```python
from build123d import *

# Parameters (mm, degrees)
SKETCH_1_W          = 260
SKETCH_1_H          = 300
EXTRUDE_1_DEPTH     = 10
SKETCH_2_W          = 220
SKETCH_2_H          = 260
CUT_EXTRUDE_1_DEPTH = 2
M3X0_51_D           = 2.5
M3X0_51_DEPTH       = 8.5
M3X0_51_TIP         = 0.751075774
SKETCH_9_W          = 260
SKETCH_9_H          = 300
SKETCH_9_W_2        = 240
SKETCH_9_H_2        = 280
CUT_EXTRUDE_3_DEPTH = 7
SKETCH_10_R         = 8
CUT_EXTRUDE_4_DEPTH = 11


with BuildPart() as part:
    # Эскиз1 → Бобышка-Вытянуть1 (new body)
    with BuildSketch(Plane(origin=(0, 0, 0), x_dir=(1, 0, 0), z_dir=(0, 1, 0))):
        Rectangle(SKETCH_1_W, SKETCH_1_H)
    extrude(amount=EXTRUDE_1_DEPTH)

    # Эскиз2 → Вырез-Вытянуть1 (cut)
    with BuildSketch(Plane.XZ):
        Rectangle(SKETCH_2_W, SKETCH_2_H)
    extrude(amount=-CUT_EXTRUDE_1_DEPTH, mode=Mode.SUBTRACT)

    # Отверстие обработанное метчиком M3x0.51
    with Locations(Plane(origin=(0, 0, 0), x_dir=(-1, 0, 0), z_dir=(0, -1, 0))):
        with Locations((-115, 135), (0, 135), (115, 135), (115, -135), (0, -135), (-115, -135), (115, 0), (-115, 0)):
            Hole(M3X0_51_D / 2, depth=M3X0_51_DEPTH)
            with Locations((0, 0, -(M3X0_51_DEPTH + M3X0_51_TIP / 2))):  # 118° drill point
                Cone(0, M3X0_51_D / 2, M3X0_51_TIP, mode=Mode.SUBTRACT)

    # Эскиз9 → Вырез-Вытянуть3 (cut)
    with BuildSketch(Plane.XZ):
        Rectangle(SKETCH_9_W, SKETCH_9_H)
        Rectangle(SKETCH_9_W_2, SKETCH_9_H_2, mode=Mode.SUBTRACT)
    extrude(amount=-CUT_EXTRUDE_3_DEPTH, mode=Mode.SUBTRACT)

    # Эскиз10 → Вырез-Вытянуть4 (cut, through all)
    with BuildSketch(Plane(origin=(0, 10, 0), x_dir=(1, 0, 0), z_dir=(0, 1, 0))):
        with Locations((74.221236429, -61.829520648)):
            Circle(SKETCH_10_R)
        with Locations((54.721236429, -61.829520648)):
            Circle(SKETCH_10_R)
        with Locations((35.221236429, -61.829520648)):
            Circle(SKETCH_10_R)
        with Locations((15.721236429, -61.829520648)):
            Circle(SKETCH_10_R)
        with Locations((-3.778763571, -61.829520648)):
            Circle(SKETCH_10_R)
        with Locations((-23.278763571, -61.829520648)):
            Circle(SKETCH_10_R)
        with Locations((-42.778763571, -61.829520648)):
            Circle(SKETCH_10_R)
        with Locations((-62.278763571, -61.829520648)):
            Circle(SKETCH_10_R)
        with Locations((27.756724611, -92.443317545)):
            Circle(SKETCH_10_R)
        with Locations((8.956724611, -92.443317545)):
            Circle(SKETCH_10_R)
        with Locations((-9.843275389, -92.443317545)):
            Circle(SKETCH_10_R)
        with Locations((-28.643275389, -92.443317545)):
            Circle(SKETCH_10_R)
        with Locations((40.197994593, -15.695954372)):
            Circle(SKETCH_10_R)
        with Locations((12.197994593, -15.695954372)):
            Circle(SKETCH_10_R)
        with Locations((-15.802005407, -15.695954372)):
            Circle(SKETCH_10_R)
        with Locations((-43.802005407, -15.695954372)):
            Circle(SKETCH_10_R)
        with Locations((64.84147229, 30.806375684)):
            Circle(SKETCH_10_R)
        with Locations((38.84147229, 30.806375684)):
            Circle(SKETCH_10_R)
        with Locations((12.84147229, 30.806375684)):
            Circle(SKETCH_10_R)
        with Locations((-13.15852771, 30.806375684)):
            Circle(SKETCH_10_R)
        with Locations((-39.15852771, 30.806375684)):
            Circle(SKETCH_10_R)
        with Locations((-65.15852771, 30.806375684)):
            Circle(SKETCH_10_R)
        with Locations((51.575799991, 106.283379385)):
            Circle(SKETCH_10_R)
        with Locations((25.075799991, 106.283379385)):
            Circle(SKETCH_10_R)
        with Locations((-1.424200009, 106.283379385)):
            Circle(SKETCH_10_R)
        with Locations((-27.924200009, 106.283379385)):
            Circle(SKETCH_10_R)
        with Locations((-0.103593652, 61.276056387)):
            Circle(SKETCH_10_R)
    extrude(amount=-CUT_EXTRUDE_4_DEPTH, mode=Mode.SUBTRACT)


solid = part.part
```
Can you work these out from the model? Positions are in its coordinate system, mm. A direction names the side the tool comes from. Round coordinates to 2 decimals unless told otherwise and drop trailing zeros. Loops run counter-clockwise (first coordinate to the right, second up) from the corner with the lowest first, then second, coordinate; pieces in that order, holes last. Notation, with made-up numbers: M 66.5,78.5 L 123.5,78.5 A12 cw 123.5,90.5 Z; hole C 61.25,14 d7. An arc over 180 degrees is marked long. Answer as a JSON object with one key per item and string values. Group by question number.
Q1. Imagine slicing it at C-C, the plane x = 94.5. Please give me the cut outline in (y, z).
Q2. Please list where these lines run through material, in increasing order: L1, parallel to Z at x = 115, y = 4.5; L2, parallel to X at y = 1, z = 80.5; L3, parallel to Z at x = -11, y = 2.75.
Q3. On a 3-axis mill with a long thin cutter (end or side, diameter ignored), from which of +Z, -Z, +X, -X, +Y, -Y can I reach the whole of each face in a straight line? I mean faces 4 (the flat face through (-2, 2, 2)), 5 (the cylindrical face through (49.842, 6.056, -98.474)). Say none if no direction works.
Q4. Will these pins go through, and if not, where does the flat tip stop? pin 1 (21 mm diameter, centred on x = 27.76, z = 92.44, fed in from -Y); pin 2 (1 mm diameter, centred on y = 1, z = 0, fed in from -X); pin 3 (6 mm diameter, centred on x = -68, y = 2, fed in from +Z); pin 4 (18.5 mm diameter, centred on x = -23.28, z = 61.83, fed in from +Y).
Q5. Imagine slicing it at A-A, the plane x = -65. Please give me the cut outline in (y, z).
Q6. We'd pull the mould along X, two halves only. Please class faces 1 (the cylindrical face through (11.8, 6.06, -38.74)), 2 (the flat face through (-2, 3, 140)), 3 (the flat face through (120, 3, -2)): +X half, -X half, draft (parallel to the pull), parting line (faces both ways), or undercut.
Q7. Imagine slicing it at B-B, the plane z = 124. Please give me the cut outline in (x, y), then the cut area to 3 significant figures.
Findings:
{
 "1": {"outline": "M 0,-140 L 7,-140 L 7,-150 L 10,-150 L 10,150 L 7,150 L 7,140 L 0,140 L 0,130 L 2,130 L 2,-130 L 0,-130 Z"},
 "2": {"L1": "z = -140 to -136.25, -133.75 to -1.25, 1.25 to 133.75, 136.25 to 140", "L2": "x = -120 to -110, 110 to 120", "L3": "z = -140 to -38.51, -23.1 to 9.3, 22.09 to 58.39, 65.27 to 84.53, 100.36 to 140"},
 "3": {"face 4": "-Y", "face 5": "+Y, -Y"},
 "4": {"pin 1": "stops at y = 2", "pin 2": "stops at x = -120", "pin 3": "stops at z = 140", "pin 4": "stops at y = 10"},
 "5": {"outline": "M 0,-140 L 7,-140 L 7,-150 L 10,-150 L 10,-38.8 L 2,-38.8 L 2,-130 L 0,-130 Z; M 0,130 L 2,130 L 2,69.35 L 10,69.35 L 10,150 L 7,150 L 7,140 L 0,140 Z; M 2,-22.81 L 10,-22.81 L 10,54.31 L 2,54.31 Z"},
 "6": {"face 1": "undercut", "face 2": "draft", "face 3": "+X half"},
 "7": {"outline": "M -130,7 L -120,7 L -120,0 L -110,0 L -110,2 L 110,2 L 110,0 L 120,0 L 120,7 L 130,7 L 130,10 L -130,10 Z", "area": "2,020 mm2"}
}
